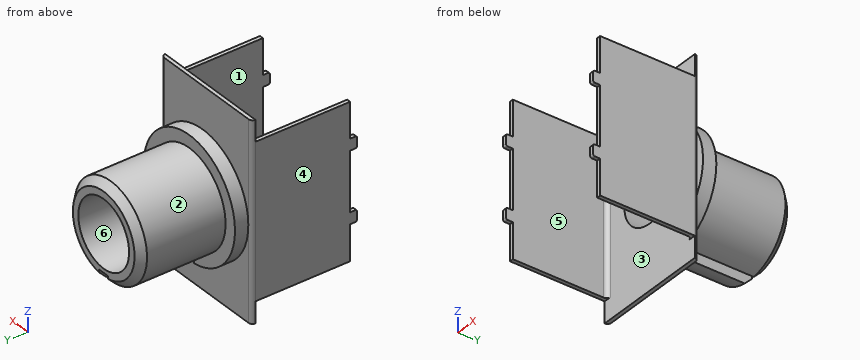
Autodesk Inventor part; units mm, degrees
ref_plane "1_XY" through (0, 5.6896, 0) normal (0, 1, 0) x (1, 0, 0)
ref_plane "1_YZ" through (0, 5.6896, 0) normal (1, 0, 0) x (0, 0, -1)
ref_plane "1_ZX" through (0, 5.6896, 0) normal (0, 0, -1) x (0, 1, 0)
sketch "Sketch_1" plane through (0, 0, 0) normal (0, 0, 1) x (1, 0, 0)
  line L0 (-3.9497, 0) -> (-3.9497, -6.7945)
  line L1 (-3.9497, -6.7945) -> (-3.6957, -6.7945)
  line L2 (-3.6957, -6.7945) -> (-3.6957, -0.254)
  arc A0 (-3.4417, 0) -> (-3.6957, -0.254) centre (-3.4417, -0.254) ccw
  line L3 (-3.4417, 0) -> (3.4417, 0)
  arc A1 (3.6957, -0.254) -> (3.4417, 0) centre (3.4417, -0.254) ccw
  line L4 (3.6957, -0.254) -> (3.6957, -6.7945)
  line L5 (3.6957, -6.7945) -> (3.9497, -6.7945)
  line L6 (3.9497, -6.7945) -> (3.9497, 0)
  arc A2 (3.9497, 0) -> (3.6957, 0.254) centre (3.6957, 0) ccw
  line L7 (3.6957, 0.254) -> (-3.6957, 0.254)
  arc A3 (-3.6957, 0.254) -> (-3.9497, 0) centre (-3.6957, 0) ccw
extrude "Extrusion1" add sketch "Sketch_1" along normal mid plane 13.0048
sketch "Sketch_2" plane through (0, 0, 0) normal (1, 0, 0) x (0, 1, 0)
  line L0 (0, 7.8029) -> (-9.398, 7.8029)
  line L1 (-9.398, 7.8029) -> (-9.398, -7.8029)
  line L2 (-9.398, -7.8029) -> (0, -7.8029)
  line L3 (0, -7.8029) -> (0, -5.0927)
  line L4 (0, -5.0927) -> (-6.3246, -5.0927)
  line L5 (-6.3246, -5.0927) -> (-6.3246, -2.7305)
  line L6 (-6.3246, -2.7305) -> (-6.6675, -2.7305)
  arc A0 (-6.7945, -2.6035) -> (-6.6675, -2.7305) centre (-6.6675, -2.6035) ccw
  line L7 (-6.7945, -2.6035) -> (-6.7945, -2.0955)
  arc A1 (-6.6675, -1.9685) -> (-6.7945, -2.0955) centre (-6.6675, -2.0955) ccw
  line L8 (-6.6675, -1.9685) -> (-6.3246, -1.9685)
  line L9 (-6.3246, -1.9685) -> (-6.3246, 1.9685)
  line L10 (-6.3246, 1.9685) -> (-6.6675, 1.9685)
  arc A2 (-6.7945, 2.0955) -> (-6.6675, 1.9685) centre (-6.6675, 2.0955) ccw
  line L11 (-6.7945, 2.0955) -> (-6.7945, 2.6035)
  arc A3 (-6.6675, 2.7305) -> (-6.7945, 2.6035) centre (-6.6675, 2.6035) ccw
  line L12 (-6.6675, 2.7305) -> (-6.3246, 2.7305)
  line L13 (-6.3246, 2.7305) -> (-6.3246, 5.0927)
  line L14 (-6.3246, 5.0927) -> (0, 5.0927)
  line L15 (0, 5.0927) -> (0, 7.8029)
extrude "Extrusion2" cut sketch "Sketch_2" along normal mid plane 7.8994
sketch "Sketch_6" plane through (0, 0, 0) normal (0, 0, 1) x (1, 0, 0)
  line L0 (0, 0.127) -> (0, 7.112)
  line L1 (0, 7.112) -> (2.7026, 7.112)
  line L2 (2.7026, 7.112) -> (3.175, 6.6396)
  line L3 (3.175, 6.6396) -> (3.175, 1.397)
  line L4 (3.175, 1.397) -> (4.0005, 1.397)
  line L5 (4.0005, 1.397) -> (4.0005, 0.508)
  line L6 (4.0005, 0.508) -> (2.3495, 0.508)
  line L7 (2.3495, 0.508) -> (2.3495, 0.127)
  line L8 (2.3495, 0.127) -> (0, 0.127)
  line L9 (0, 0.127) -> (0, 7.112)
revolve "Revolution1" add sketch "Sketch_6" angle 360 about axis through (0, 0.127, 0) along (0, -1, 0)
thread "Thread1"
sketch "Sketch_8" plane through (0, 0.254, 0) normal (0, 1, 0) x (1, 0, 0)
  line L0 (-0.3937, 2.4892) -> (0.3937, 2.4892)
  line L1 (0.3937, 2.4892) -> (0.3937, 10.4902)
  line L2 (0.3937, 10.4902) -> (-0.3937, 10.4902)
  line L3 (-0.3937, 10.4902) -> (-0.3937, 2.4892)
extrude "Extrusion3" cut sketch "Sketch_8" along normal blind 7.8232
sketch "Sketch_10_ALT_Drilling_1" plane through (0, 0, 0) normal (0, 0, 1) x (1, 0, 0)
  line L0 (0, 0) -> (0, 7.747)
  line L1 (0, 7.747) -> (2.2225, 7.747)
  line L2 (2.2225, 7.747) -> (2.2225, 0)
  line L3 (2.2225, 0) -> (0, 0)
  line L4 (0, 0) -> (0, 7.747)
revolve "Revolution2" cut sketch "Sketch_10_ALT_Drilling_1" angle 360 about axis through (0, 0, 0) along (0, -1, 0)
ref_plane "1_XY" through (0, 5.6896, 0) normal (0, 1, 0) x (1, 0, 0)
ref_plane "1_YZ" through (0, 5.6896, 0) normal (1, 0, 0) x (0, 0, -1)
ref_plane "1_ZX" through (0, 5.6896, 0) normal (0, 0, -1) x (0, 1, 0)
ref_plane "2_XY" through (0, 4.2672, 0) normal (0, 1, 0) x (1, 0, 0)
ref_plane "2_YZ" through (0, 4.2672, 0) normal (1, 0, 0) x (0, 0, -1)
ref_plane "2_ZX" through (0, 4.2672, 0) normal (0, 0, -1) x (0, 1, 0)
ref_plane "3_XY" through (0, 2.8448, 0) normal (0, 1, 0) x (1, 0, 0)
ref_plane "3_YZ" through (0, 2.8448, 0) normal (1, 0, 0) x (0, 0, -1)
ref_plane "3_ZX" through (0, 2.8448, 0) normal (0, 0, -1) x (0, 1, 0)
ref_plane "4_XY" through (0, 1.778, 0) normal (0, 1, 0) x (1, 0, 0)
ref_plane "4_YZ" through (0, 1.778, 0) normal (1, 0, 0) x (0, 0, -1)
ref_plane "4_ZX" through (0, 1.778, 0) normal (0, 0, -1) x (0, 1, 0)
ref_plane "to_base_XY" through (0, 0, 0) normal (0, 1, 0) x (1, 0, 0)
ref_plane "to_base_YZ" through (0, 0, 0) normal (1, 0, 0) x (0, 0, -1)
ref_plane "to_base_ZX" through (0, 0, 0) normal (0, 0, -1) x (0, 1, 0)
properties part number "M201A1M201BR-bushing"
Check sheet for the modelled part. Datum: model origin and axes. Units: mm. Face numbers are marked on the shaded views. A direction names the side the tool comes from. Round coordinates to 2 decimals unless told otherwise and drop trailing zeros. Order: outer loops, then holes, each group sorted by start corner. A loop starts at its lowest first (then second) coordinate and runs counter-clockwise, first axis right, second up.
1) Section check B-B (y = -2.5). Record the boundary of the cut face in (x, z).
2) Scan lines: line 1 (Z direction, x = 0, y = 2.75) (1 decimal); line 2 (Y direction, x = 0.5, z = 2.5); line 3 (X direction, y = -1.75, z = -3.25). Record each from-to range of solid material in increasing order.
3) Tool access check on the marked faces 5 and 6. Record the directions out of +Z, -Z, +X, -X, +Y, -Y that give a thin tool (end or side, any length) a straight path to the whole face; none if there is none.
4) Mould release check, pull along X, two halves, no side actions. Record for the marked faces 1, 2, 3 and 4: +X half, -X half, draft (parallel to the pull), parting line (faces both ways), or undercut.
5) Go/stop test with flat-tipped pins: pin 1 Ø2 at (x, z) = (-1.5, -2.5) entering from +Y; pin 2 Ø3 at (y, z) = (3.5, 3.5) entering from -X; pin 3 Ø1 at (x, y) = (-1, 3.5) entering from -Z; pin 4 Ø3 at (x, z) = (2.5, 5) entering from +Y. Record where each tip stops, or that it passes through.
Result:
1. outline: (-3.95, -5.09) - (-3.7, -5.09) - (-3.7, 5.09) - (-3.95, 5.09) - close; (3.7, -5.09) - (3.95, -5.09) - (3.95, 5.09) - (3.7, 5.09) - close
2. line 1: z = -2.5 to -2.2, 2.2 to 3.2
2. line 2: y = 0 to 0.25, 0.51 to 7.11
2. line 3: x = -3.95 to -3.7, 3.7 to 3.95
3. face 5: +Z, -Z, -Y
3. face 6: +Y, -Y
4. face 1: undercut
4. face 2: parting line
4. face 3: undercut
4. face 4: -X half
5. pin 1: stops at y = 7.11
5. pin 2: stops at x = -2.47
5. pin 3: stops at z = -3.14
5. pin 4: stops at y = 0.25
